Part model, mm, in its own coordinate system. A direction names the side the tool comes from. Round coordinates to 2 decimals unless told otherwise and drop trailing zeros. Loops run counter-clockwise (first coordinate to the right, second up) from the corner with the lowest first, then second, coordinate; pieces in that order, holes last.
Autodesk Inventor part; units mm, degrees
ref_plane "YZ Plane" through (0, 0, 0) normal (1, 0, 0) x (0, 1, 0)
ref_plane "XZ Plane" through (0, 0, 0) normal (0, 1, 0) x (-1, 0, 0)
ref_plane "XY Plane" through (0, 0, 0) normal (0, 0, 1) x (1, 0, 0)
sketch "Sketch1" plane through (0, 0, 0) normal (0, 0, 1) x (1, 0, 0)
  arc A0 (0, -19.05) -> (19.05, 0) centre (0, 0) ccw
  arc A1 (-12.7, 0) -> (12.7, 0) centre (0, 0) ccw
  line L0 (-19.05, 0) -> (19.05, 0) construction
  line L1 (-19.05, 0) -> (-19.05, -19.05)
  line L2 (-19.05, -19.05) -> (0, -19.05)
  line L3 (-19.05, 0) -> (-12.7, 0)
  line L4 (12.7, 0) -> (19.05, 0)
  circle A2 centre (0, 0) radius 19.05 construction
  dimension "d0" = 38.1
  dimension "d1" = 25.4
extrude "Extrusion1" add sketch "Sketch1" along normal mid plane 3.81
sketch "Sketch2" plane through (0, 0, 0) normal (0, 0, 1) x (1, 0, 0)
  line L0 (-19.05, 0) -> (-12.7, 0)
  line L1 (-19.05, -19.05) -> (-19.05, 0)
  line L2 (-19.05, 0) -> (-19.05, 10.9985)
  line L3 (-19.05, 10.9985) -> (-12.7, 0)
  line L4 (-12.7, 0) -> (-19.05, 0)
  point P0 (0, 0)
  dimension "d5" = 60
extrude "Extrusion2" add sketch "Sketch2" along normal mid plane 3.81
properties part number "hook"
1) Drop flat-ended pins along their axis: pin 1 Ø1.5 at (y, z) = (-1.5, -1) entering from +X; pin 2 Ø2 at (x, z) = (12.5, 1) entering from +Y; pin 3 Ø1 at (x, z) = (-4.5, 1) entering from +Y. Give the stop position or say it passes through.
Values:
pin 1: stops at x = 19.04
pin 2: stops at y = 0
pin 3: stops at y = -11.67
2) Slice it at A-A, the plane z = 1.25. Give the cut face in (x, y), then the cut area to 3 significant figures.
Values:
outline: (-19.05, -19.05) - (0, -19.05) arc R19.05 ccw to (19.05, 0) - (12.7, 0) arc R12.7 cw to (-12.7, 0) - (-19.05, 11) - close
area: 429 mm2
3) Wall check: line 1 along X through (y, z) = (-5, -1.55); line 2 along X through (y, z) = (-2, -0.1); line 3 along Y through (x, z) = (-16, -1.45). Give the ranges that are in metal, low to high.
Values:
line 1: x = -19.05 to -11.67, 11.67 to 18.38
line 2: x = -19.05 to -12.54, 12.54 to 18.94
line 3: y = -19.05 to 5.72
4) Slice it at C-C, the plane x = 16. Give the cut face in (y, z) (3 decimals).
Values:
outline: (-10.339, -1.905) - (0, -1.905) - (0, 1.905) - (-10.339, 1.905) - close
5) Tool access for faces 1 (the face through (-10, -19.05, 0)), 2 (the face through (16, 0, 0)): list every direction of +Z, -Z, +X, -X, +Y, -Y with a clear straight run to the whole face (end or side of a thin tool).
Values:
face 1: +Z, -Z, +X, -X, -Y
face 2: +Z, -Z, +X, +Y
6) Slice it at B-B, the plane y = 8.5. Give the cut face in (x, z) (3 decimals), then the cut area to 3 significant figures.
Values:
outline: (-19.05, -1.905) - (-17.607, -1.905) - (-17.607, 1.905) - (-19.05, 1.905) - close
area: 5.50 mm2
7) Mould opens along X. For faces 3 (the face through (0.279, -12.697, -0.027)), 4 (the face through (-15.92, 5.58, -0.03)), 5 (the face through (-5, -14, -1.905)) say: released by +X, released by -X, zero draft, split by the parting line, or undercut.
Values:
face 3: undercut
face 4: released by +X
face 5: zero draft
